The listing builds one solid part. Answer for the finished solid, in the listing's coordinates (mm). Give positions to 0.01 mm unless a question says otherwise; leave off trailing zeros. Write each loop counter-clockwise with the first axis right and the second up, starting at its lowest first coordinate (ties: lowest second). Pieces come first, ordered by that corner, then holes. Notation, with made-up numbers: (47.5, 82) - (74.5, 82) arc R28 cw to (74.5, 120) - close; hole circle Ø6 at (60, 23.25). An arc over 180 degrees is marked (long way). Return JSON: item names as keys, results as strings.
from build123d import *

# Parameters (mm, degrees)
SKETCH1_W               = 475.54896
SKETCH1_H               = 625.48516
BASE_FLANGE1_DEPTH      = 3.175
CUT_EXTRUDE1_DEPTH      = 393.880013884
CUT_EXTRUDE1_DEPTH_BACK = 393.880013884
SKETCH2_W               = 60.325
SKETCH2_H               = 3.175
SKETCH3_W               = 107.287119944
SKETCH3_H               = 30.1625
SKETCH3_W_2             = 34.47288
SKETCH3_H_2             = 111.597499944
SKETCH3_W_3             = 27.86888
BOSS_EXTRUDE1_DEPTH     = 3.175


# Sheet-metal steps are written as plain solids
with BuildPart() as part:
    # Sketch1 → Base-Flange1 (new body)
    with BuildSketch(Plane.XY):
        Rectangle(SKETCH1_W, SKETCH1_H)
    extrude(amount=-BASE_FLANGE1_DEPTH)

    # Sketch2 → Cut-Extrude1 (cut, two sides: drawn at the far end of the back side and taken through both)
    with BuildSketch(Plane.XY.offset(-CUT_EXTRUDE1_DEPTH_BACK)):
        with Locations((-186.97448, 96.52)):
            Rectangle(SKETCH2_W, SKETCH2_H)
        with Locations((-186.97448, 0)):
            Rectangle(SKETCH2_W, SKETCH2_H)
        with Locations((186.97448, 0)):
            Rectangle(SKETCH2_W, SKETCH2_H)
        with Locations((186.97448, 96.52)):
            Rectangle(SKETCH2_W, SKETCH2_H)
        with Locations((-186.97448, 193.04)):
            Rectangle(SKETCH2_W, SKETCH2_H)
        with Locations((186.97448, 193.04)):
            Rectangle(SKETCH2_W, SKETCH2_H)
        with Locations((-186.97448, -96.52)):
            Rectangle(SKETCH2_W, SKETCH2_H)
        with Locations((186.97448, -96.52)):
            Rectangle(SKETCH2_W, SKETCH2_H)
        with Locations((-186.97448, -193.04)):
            Rectangle(SKETCH2_W, SKETCH2_H)
        with Locations((186.97448, -193.04)):
            Rectangle(SKETCH2_W, SKETCH2_H)
    extrude(amount=CUT_EXTRUDE1_DEPTH + CUT_EXTRUDE1_DEPTH_BACK, mode=Mode.SUBTRACT)

    # Sketch3 → Boss-Extrude1 (add)
    with BuildSketch(Plane.XY):
        with Locations((184.130920028, 327.82383)):
            Rectangle(SKETCH3_W, SKETCH3_H)
        with Locations((-255.01092, 256.943830028)):
            Rectangle(SKETCH3_W_2, SKETCH3_H_2)
        with Locations((-251.70892, -256.943830028)):
            Rectangle(SKETCH3_W_3, SKETCH3_H_2)
        with Locations((184.130920028, -327.82383)):
            Rectangle(SKETCH3_W, SKETCH3_H)
    extrude(amount=-BOSS_EXTRUDE1_DEPTH)


solid = part.part
Item 1: A cutting plane is placed at C-C on y = -118. Determine the outline of the cut face in (x, z) (3 decimals), then the cut area to 3 significant figures.
Answer below:
{"outline": "(-237.774, -3.175) - (237.774, -3.175) - (237.774, 0) - (-237.774, 0) - close", "area": "1,510 mm²"}
Item 2: Consider L1, parallel to Y at x = -186, z = -2.35; L2, parallel to Y at x = 171.5, z = -1.65; L3, parallel to Y at x = 73.5, z = -2.35. Determine where each line is inside the solid, lowest interval first.
Answer below:
{"L1": "y = -312.74 to -194.63, -191.45 to -98.11, -94.93 to -1.59, 1.59 to 94.93, 98.11 to 191.45, 194.63 to 312.74", "L2": "y = -342.91 to -194.63, -191.45 to -98.11, -94.93 to -1.59, 1.59 to 94.93, 98.11 to 191.45, 194.63 to 342.91", "L3": "y = -312.74 to 312.74"}
Item 3: A cutting plane is placed at B-B on z = -0.5. Give the number of separate pieces and of enclosed holes in the cut face, then the cut area to 3 significant figures.
Answer below:
{"separate pieces": "1", "enclosed holes": "10", "area": "309,000 mm²"}
Item 4: A cutting plane is placed at A-A on x = -197. Determine the outline of the cut face in (y, z) (1 decimal).
Answer below:
{"outline": "(-312.7, -3.2) - (-194.6, -3.2) - (-194.6, 0) - (-312.7, 0) - close; (-191.5, -3.2) - (-98.1, -3.2) - (-98.1, 0) - (-191.5, 0) - close; (-94.9, -3.2) - (-1.6, -3.2) - (-1.6, 0) - (-94.9, 0) - close; (1.6, -3.2) - (94.9, -3.2) - (94.9, 0) - (1.6, 0) - close; (98.1, -3.2) - (191.5, -3.2) - (191.5, 0) - (98.1, 0) - close; (194.6, -3.2) - (312.7, -3.2) - (312.7, 0) - (194.6, 0) - close"}
Item 5: Flat-ended cylindrical pins translate along their axes: P1, Ø1, axis at y = -192.5, z = -1, coming from the -X side; P2, Ø1, axis at x = -172, z = -1.5, coming from the -Y side; P3, Ø1, axis at y = -274.5, z = -1.5, coming from the -X side. Find the tip coordinate at first contact, or state that the pin passes through.
Answer below:
{"P1": "stops at x = -237.77", "P2": "stops at y = -312.74", "P3": "stops at x = -265.64"}
